Autodesk Inventor part; units mm, degrees
ref_plane "YZ Plane" through (0, 0, 0) normal (1, 0, 0) x (0, 1, 0)
ref_plane "XZ Plane" through (0, 0, 0) normal (0, 1, 0) x (-1, 0, 0)
ref_plane "XY Plane" through (0, 0, 0) normal (0, 0, 1) x (1, 0, 0)
sketch "Sketch1" plane through (0, 0, 0) normal (0, 1, 0) x (-1, 0, 0)
  circle A0 centre (0, 0) radius 82.55
  circle A1 centre (0, 0) radius 88.9
  dimension "d0" = 165.1
  dimension "d1" = 177.8
extrude "Extrusion1" add sketch "Sketch1" along normal blind 50.8
sketch "Sketch2" plane through (0, 0, 0) normal (0, -1, 0) x (1, 0, 0)
  arc A0 (40.4112, 58.3717) -> (58.3717, 40.4112) centre (49.3914, 49.3914) ccw
  arc A1 (58.3717, -40.4112) -> (40.4112, -58.3717) centre (49.3914, -49.3914) ccw
  arc A2 (-40.4112, -58.3717) -> (-58.3717, -40.4112) centre (-49.3914, -49.3914) ccw
  arc A3 (-58.3717, 40.4112) -> (-40.4112, 58.3717) centre (-49.3914, 49.3914) ccw
  circle A4 centre (0, 0) radius 82.55
  line L0 (-40.4112, 58.3717) -> (-48.6965, 66.657)
  line L1 (-58.3717, 40.4112) -> (-66.657, 48.6965)
  line L2 (58.3717, 40.4112) -> (66.657, 48.6965)
  line L3 (40.4112, 58.3717) -> (48.6965, 66.657)
  line L4 (58.3717, -40.4112) -> (66.657, -48.6965)
  line L5 (40.4112, -58.3717) -> (48.6965, -66.657)
  line L6 (-40.4112, -58.3717) -> (-48.6965, -66.657)
  line L7 (-58.3717, -40.4112) -> (-66.657, -48.6965)
  dimension "d4" = 25.4
extrude "Extrusion2" add sketch "Sketch2" against normal blind 6.35 contours L3 A4 L2 A0 | L0 A3 L1 A4 | A4 L5 A1 L4 | L7 A2 L6 A4
properties part number "aluminumMount" material "Aluminum 6061-AHC"
Here's how the part is built. I have some questions about the finished solid (model axes, mm). A direction names the side the tool comes from. Round coordinates to 2 decimals unless told otherwise and drop trailing zeros. Loops run counter-clockwise (first coordinate to the right, second up) from the corner with the lowest first, then second, coordinate; pieces in that order, holes last. Notation, with made-up numbers: M 19.5,6.25 L 27.5,6.25 A5 cw 27.5,13.25 Z; hole C 68,18 d1. An arc over 180 degrees is marked long. Write each question's results on one line, items separated by ' | '. Start each with the question number.
(1) If I drill on probe 1 along Z at (x, y) = (1, 24.5); probe 2 along X at (y, z) = (7.5, 75.5); probe 3 along X at (y, z) = (48.5, -39.5), over which ranges is the centre line in solid material (lowest first)? Write a range as from..to.
(2) I want a section at A-A (x = 0). Please give me the cut outline in (y, z), then the cut area to 3 significant figures.
(3) I want a section at C-C (y = 26). Please give me the cut outline in (x, z).
(4) Will these pins go through, and if not, where does the flat tip stop? P1, Ø8, axis at y = 6.5, z = -13, coming from the -X side; P2, Ø24, axis at x = -51, z = -44.5, coming from the +Y side; P3, Ø4, axis at x = -10, y = 12.5, coming from the -Z side.
(5) I want a section at B-B (z = 0). Please give me the cut outline in (x, y), then the cut area to 3 significant figures.
(6) Thinking about a two-plate mould opening in X: for faces 4 (the flat face through (-26, 50.8, -79)), 5 (the flat face through (-62.46, 3.13, -44.5)), 6 (the cylindrical face through (-84.795, 25.044, -26.703)), which applies, pulls with the +X half, pulls with the -X half, needs draft (parallel to the pull), parting line crosses it, or undercut?
(7) On a 3-axis mill with a long thin cutter (end or side, diameter ignored), from which of +Z, -Z, +X, -X, +Y, -Y can I reach the whole of each face in a straight line? I mean faces 1 (the flat face through (-39, 0, 47)), 2 (the flat face through (-49, 6.35, 49)), 3 (the flat face through (44.5, 3.13, -62.46)). Say none if no direction works.
Solved:
1) probe 1: z = -88.89..-82.54, 82.54..88.89 | probe 2: x = -46.94..-33.38, 33.38..46.94 | probe 3: x = -79.64..-72.49, 72.49..79.64
2) outline: M 0,-88.9 L 50.8,-88.9 L 50.8,-82.55 L 0,-82.55 Z; M 0,82.55 L 50.8,82.55 L 50.8,88.9 L 0,88.9 Z | area: 645 mm²
3) outline: C 0,0 d177.8; hole C 0,0 d165.1
4) P1: stops at x = -88.44 | P2: stops at y = 6.35 | P3: stops at z = -88.54
5) outline: M -88.9,0 L -82.55,0 L -82.55,50.8 L -88.9,50.8 Z; M 82.55,0 L 88.9,0 L 88.9,50.8 L 82.55,50.8 Z | area: 645 mm²
6) face 4: needs draft | face 5: undercut | face 6: parting line crosses it
7) face 1: +Z, -Z, +X, -X, -Y | face 2: +Y | face 3: +Y, -Y
